```python
from build123d import *

# Parameters (mm, degrees)
SKETCH007_W     = 127
SKETCH007_H     = 28
PAD003_DEPTH    = 6.8
SKETCH008_W     = 1.5
SKETCH008_H     = 6.8
PAD004_DEPTH    = 1.5
SKETCH010_W     = 1.5
SKETCH010_H     = 6.8
PAD005_DEPTH    = 1.5
SKETCH012_R     = 3.03
POCKET004_DEPTH = 6.801
SKETCH013_R     = 1.05
SKETCH013_R_2   = 1.5
POCKET005_DEPTH = 29.501
SKETCH014_W     = 101
SKETCH014_H     = 5.7
POCKET006_DEPTH = 1.69
SKETCH021_W     = 7
SKETCH021_H     = 3.4
PAD009_DEPTH    = 7


with BuildPart() as part:
    # Sketch007 → Pad003 (new body)
    with BuildSketch(Plane(origin=(0.865, 0, 0), x_dir=(1, 0, 0), z_dir=(0, 0, 1))):
        with Locations((-63.932219, -3.966905)):
            Rectangle(SKETCH007_W, SKETCH007_H)
    extrude(amount=PAD003_DEPTH)

    # Sketch008 → Pad004 (new body)
    with BuildSketch(Plane(origin=(0.865, -17.966905, 0), x_dir=(1, 0, 0), z_dir=(0, -1, 0))):
        with Locations((-126.682219, 3.4)):
            Rectangle(SKETCH008_W, SKETCH008_H)
    extrude(amount=PAD004_DEPTH)

    # Sketch010 → Pad005 (new body)
    with BuildSketch(Plane(origin=(0.865, 10.033095, 0), x_dir=(-1, 0, 0), z_dir=(0, 1, 0))):
        with Locations((126.682219, 3.4)):
            Rectangle(SKETCH010_W, SKETCH010_H)
    extrude(amount=PAD005_DEPTH)

    # Sketch012 → Pocket004 (cut, through all)
    with BuildSketch(Plane(origin=(0.865, 0, 6.8), x_dir=(1, 0, 0), z_dir=(0, 0, 1))):
        with Locations((-56.432219, -3.966905)):
            Circle(SKETCH012_R)
    extrude(amount=-POCKET004_DEPTH, mode=Mode.SUBTRACT)

    # Sketch013 → Pocket005 (cut, through all)
    with BuildSketch(Plane(origin=(0.865, -17.966905, 0), x_dir=(1, 0, 0), z_dir=(0, -1, 0))):
        with Locations((-56.432219, 3.4)):
            Circle(SKETCH013_R)
        with Locations((-117.432219, 3.4)):
            Circle(SKETCH013_R_2)
        with Locations((-34.475986, 3.4)):
            Circle(SKETCH013_R_2)
    extrude(amount=-POCKET005_DEPTH, mode=Mode.SUBTRACT)

    # Sketch014 → Pocket006 (cut)
    with BuildSketch(Plane(origin=(0.865, 0, 0), x_dir=(1, 0, 0), z_dir=(0, 0, -1))):
        with Locations((-50.932219, 11.516905)):
            Rectangle(SKETCH014_W, SKETCH014_H)
    extrude(amount=-POCKET006_DEPTH, mode=Mode.SUBTRACT)

    # Sketch021 → Pad009 (new body)
    with BuildSketch(Plane.YZ.offset(0.432781)):
        with Locations((-3.966905, 1.7)):
            Rectangle(SKETCH021_W, SKETCH021_H)
    extrude(amount=PAD009_DEPTH)


solid = part.part
```
The model under review builds one solid part; all positions refer to its coordinate system, in mm. A direction names the side the tool comes from. Coordinates: 2 decimals unless noted, no trailing zeros. Write each loop counter-clockwise with the first axis right and the second up, starting at its lowest first coordinate (ties: lowest second). Pieces come first, ordered by that corner, then holes. Notation, with made-up numbers: (61.5, 23) - (98.5, 23) arc R23 cw to (98.5, 61) - close; hole circle Ø8 at (-9.75, 43). An arc over 180 degrees is marked (long way). Answer in a Markdown table with one row per item. Add a question column.
Q1. Consider section C-C on x = -107. Give the boundary of the cut face in (y, z), then the cut area to 3 significant figures.
Q2. Consider section A-A on y = 5. Give the boundary of the cut face in (x, z), then the cut area to 3 significant figures.
Q3. Clearance check with flat-ended pins moving along their axes: pin 1 (3.5 mm diameter, centred on x = -116.57, z = 3.4, fed in from -Y); pin 2 (1.2 mm diameter, centred on y = 11, z = 4, fed in from +X); pin 3 (1.7 mm diameter, centred on x = 5, z = 1.5, fed in from -Y); pin 4 (12 mm diameter, centred on x = -66.5, y = 4, fed in from -Z). State where each tip first meets the part, or that it passes through.
Q4. Draft analysis for pull direction Z (two halves, no side actions). For faces 1 (the face through (-51, -12, 1.69)), 2 (the face through (-63, -17.967, 3)), 3 (the face through (-115.136, -4.163, 3.851)), 4 (the face through (4, -4, 3.4)), state which applies: +Z half, -Z half, draft (parallel to the pull), parting line (faces both ways), or undercut.
Q5. To check wall thickness, follow line 1 along Y through (x, z) = (-22, 0.5); line 2 along Y through (x, z) = (-111, 5); line 3 along X through (y, z) = (-8, 5.5). State the ranges of each line that lie inside material, in increasing order. Write a range as from..to.
Q6. Consider section B-B on x = -21. Give the boundary of the cut face in (y, z).
Q7. For faces 5 (the face through (4, -7.467, 2)), 6 (the face through (-59, -4, 0)), 7 (the face through (-63, 10.033, 3)), list the 3-axis set-ups (+Z, -Z, +X, -X, +Y, -Y) from which the entire face can be reached by the end or side of a thin tool; tool diameter is ignored.
Answers below:
| question | item | result |
|---|---|---|
| 1 | outline | (-17.97, 0) - (10.03, 0) - (10.03, 6.8) - (-17.97, 6.8) - close |
| 1 | area | 190 mm² |
| 2 | outline | (-126.57, 0) - (0.43, 0) - (0.43, 6.8) - (-126.57, 6.8) - close; hole circle Ø3 at (-116.57, 3.4); hole circle Ø2.1 at (-55.57, 3.4); hole circle Ø3 at (-33.61, 3.4) |
| 2 | area | 846 mm² |
| 3 | pin 1 | y = -17.97 |
| 3 | pin 2 | x = -125.07 |
| 3 | pin 3 | y = -7.47 |
| 3 | pin 4 | z = 0 |
| 4 | face 1 | -Z half |
| 4 | face 2 | draft |
| 4 | face 3 | undercut |
| 4 | face 4 | +Z half |
| 5 | line 1 | -17.97..-14.37, -8.67..10.03 |
| 5 | line 2 | -17.97..10.03 |
| 5 | line 3 | -126.57..0.43 |
| 6 | outline | (-17.97, 0) - (-14.37, 0) - (-14.37, 1.69) - (-8.67, 1.69) - (-8.67, 0) - (10.03, 0) - (10.03, 6.8) - (-17.97, 6.8) - close |
| 7 | face 5 | +Z, -Z, +X, -Y |
| 7 | face 6 | -Z, +X, -X, +Y, -Y |
| 7 | face 7 | +Z, -Z, +X, +Y |
